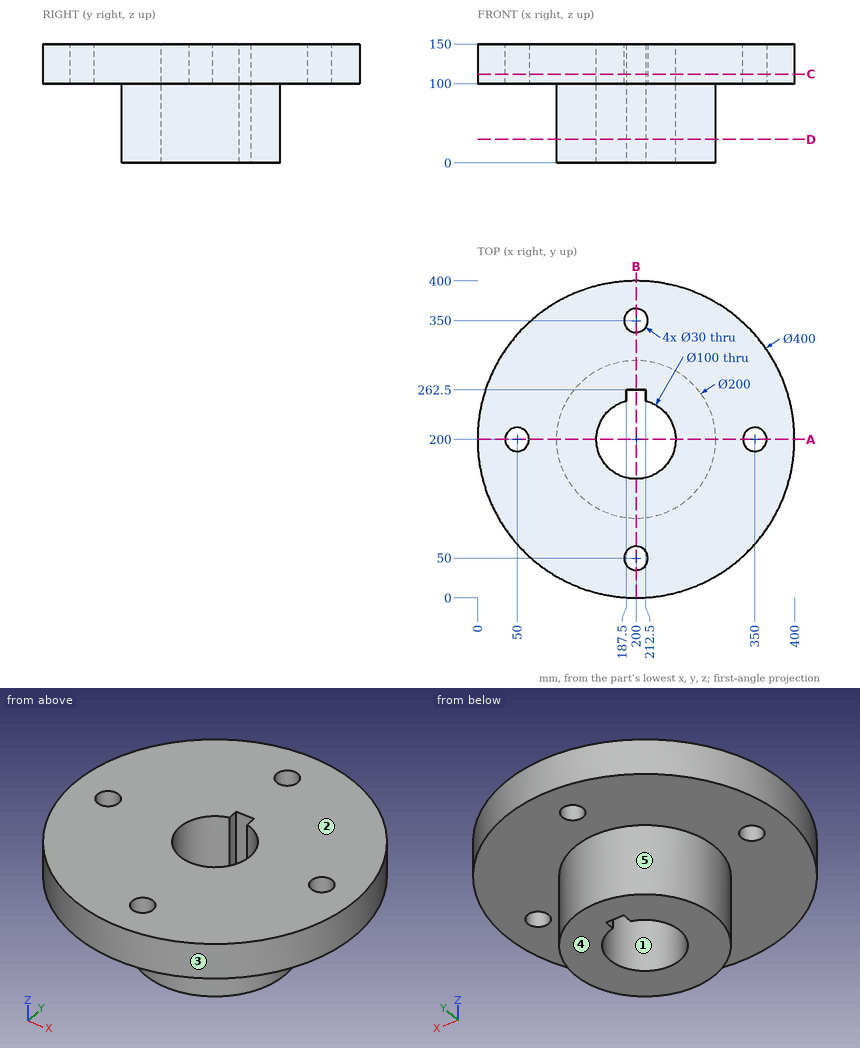
Study the drawing (mm; zero at the part's minimum x, y, z) and answer. A direction names the side the tool comes from. Coordinates: 2 decimals unless noted, no trailing zeros. Write each loop counter-clockwise with the first axis right and the second up, starting at its lowest first coordinate (ties: lowest second). Pieces come first, ordered by that corner, then holes. Notation, with made-up numbers: M 64,-40 L 105,-40 A23 ccw 105,-10 Z; hole C 85,43 d10. An arc over 180 degrees is marked long. Use one line per item in the form item = value.
Item 1: The mould has two halves that part along Y. Classify the marked faces 1, 2 and 3: released by +Y, released by -Y, zero draft, split by the parting line, or undercut.
Model answer:
face_1 = undercut
face_2 = zero draft
face_3 = split by the parting line
Item 2: Find section A-A, the plane y = 200. Give the vertices of the cut face in (x, z).
Model answer:
outline = M 0,100 L 35,100 L 35,150 L 0,150 Z; M 65,100 L 100,100 L 100,0 L 150,0 L 150,150 L 65,150 Z; M 250,0 L 300,0 L 300,100 L 335,100 L 335,150 L 250,150 Z; M 365,100 L 400,100 L 400,150 L 365,150 Z
Item 3: Given P1, Ø7, axis at y = 258, z = 40.5, coming from the +X side; P2, Ø1.5, axis at x = 139, y = 319, coming from the -Z side; P3, Ø6, axis at x = 170, z = 85.5, coming from the +Y side, each flat-ended and moving along its own axis, determine where each tip first touches the part or whether it passes through.
Model answer:
P1 = 283.84
P2 = 100
P3 = 296.29
Item 4: Find section D-D, the plane z = 29.5. Give the vertices of the cut face in (x, y).
Model answer:
outline = C 200,200 d200; hole M 187.5,248.41 A50 ccw long 212.5,248.41 L 212.5,262.5 L 187.5,262.5 Z
Item 5: Find section B-B, the plane x = 200. Give the vertices of the cut face in (y, z), plus the area to 3 significant figures.
Model answer:
outline = M 0,100 L 35,100 L 35,150 L 0,150 Z; M 65,100 L 100,100 L 100,0 L 150,0 L 150,150 L 65,150 Z; M 262.5,0 L 300,0 L 300,100 L 335,100 L 335,150 L 262.5,150 Z; M 365,100 L 400,100 L 400,150 L 365,150 Z
area = 20,100 mm2
Item 6: Find the intervals of material crossed by probe 1 along Y at (x, z) = (197, 121); probe 2 along Z at (x, y) = (157, 318); probe 3 along X at (y, z) = (244.5, 43), in increasing order.
Model answer:
probe_1 = 0.02 to 35.3, 64.7 to 150.09, 262.5 to 335.3, 364.7 to 399.98
probe_2 = 100 to 150
probe_3 = 110.45 to 177.2, 222.8 to 289.55
Item 7: For the marked faces 4 and 5, determine the directions among +Z, -Z, +X, -X, +Y, -Y from which every point of the face is accessible in a straight line to the end or side of a thin tool.
Model answer:
face_4 = -Z, +X, -X, +Y, -Y
face_5 = -Z
Item 8: Find section C-C, the plane z = 112. Give the vertices of the cut face in (x, y).
Model answer:
outline = C 200,200 d400; hole C 50,200 d30; hole C 200,50 d30; hole C 200,350 d30; hole M 187.5,248.41 A50 ccw long 212.5,248.41 L 212.5,262.5 L 187.5,262.5 Z; hole C 350,200 d30
